Geometry check sheet. Reference: the model listing, model coordinates, mm. Round coordinates to 2 decimals unless told otherwise and drop trailing zeros. Order: outer loops, then holes, each group sorted by start corner. A loop starts at its lowest first (then second) coordinate and runs counter-clockwise, first axis right, second up.
(1) Cross-section at A-A on y = -4.5. Enter the section's corners in (x, z), and give its area (3 significant figures).
(2) Draft check along Y on faces 1 (the face through (-0.187, -39.246, 0.172)), 2 (the face through (0, 43, 0)), 3 (the face through (0, -43, 0)). Enter one of: pulls with the +Y half, pulls with the -Y half, needs draft (parallel to the pull), parting line crosses it, or undercut.
(3) Gauge pin test, flat ends, axial feed: P1, Ø6, axis at y = -5.5, z = 6, coming from the +X side; P2, Ø12, axis at y = -22.5, z = 9, coming from the -X side; P3, Ø4, axis at x = 2.5, y = 22.5, coming from the -Z side; P4, Ø7.5, axis at x = 0, y = 35, coming from the +Z side. Record the tip position at first contact, or that the pin passes through.
(4) Thickness scan on L1, parallel to Z at x = -0.5, y = 26.5; L2, parallel to Y at x = -3, z = -7.5; L3, parallel to X at y = 35, z = 9. Record the ranges inside material, lowest first.
(5) Cross-section at B-B on x = 2. Count the separate pieces of the cut face and the enclosed holes in it, and give its area (3 significant figures).
(6) Cross-section at D-D on y = 35. Enter the section's corners in (x, z), and give its area (3 significant figures).
from build123d import *

# Parameters (mm, degrees)
ESBO_O1_R                = 12.5
RESSALTO_EXTRUS_O1_DEPTH = 43
CHANFRO1_SIZE            = 2
ESBO_O2_R                = 4.25
CORTE_EXTRUS_O1_DEPTH    = 43


with BuildPart() as part:
    # Esboço1 → Ressalto-extrusão1 (new, symmetric)
    with BuildSketch(Plane(origin=(0, 0, 0), x_dir=(1, 0, 0), z_dir=(0, 1, 0))):
        with Locations(Location((0, 0, 0), (0, 0, 270))):
            Circle(ESBO_O1_R)
    extrude(amount=RESSALTO_EXTRUS_O1_DEPTH, both=True)

    # Chanfro1
    chanfro1_edges = [part.edges().sort_by_distance(p)[0] for p in [
        (0, -43, -12.5),
        (0, 43, -12.5),
    ]]
    chamfer(chanfro1_edges, length=CHANFRO1_SIZE)

    # Esboço2 → Corte-extrusão1 (cut, symmetric)
    with BuildSketch(Plane.XY):
        with Locations(Location((0, 35, 0), (0, 0, 89.999999985))):
            Circle(ESBO_O2_R)
        with Locations(Location((0, -35, 0), (0, 0, 89.999999985))):
            Circle(ESBO_O2_R)
    extrude(amount=CORTE_EXTRUS_O1_DEPTH, both=True, mode=Mode.SUBTRACT)


solid = part.part
Found:
1. outline: circle Ø25 at (0, 0)
1. area: 491 mm2
2. face 1: undercut
2. face 2: pulls with the +Y half
2. face 3: pulls with the -Y half
3. P1: stops at x = 12.13
3. P2: stops at x = -12.13
3. P3: stops at z = -12.49
3. P4: passes through
4. L1: z = -12.49 to 12.49
4. L2: y = -43 to -38.01, -31.99 to 31.99, 38.01 to 43
4. L3: x = -8.67 to -4.25, 4.25 to 8.67
5. separate pieces: 3
5. enclosed holes: 0
5. area: 1,740 mm2
6. outline: (-4.25, -11.76) - (-4.25, 11.76) arc R12.5 ccw to start; (4.25, -11.76) arc R12.5 ccw to (4.25, 11.76) - close
6. area: 283 mm2
